The figure shows three views and two pictorial views of one solid part (mm, origin at its lowest corner). Answer the questions. Give positions to 0.01 mm unless a question says otherwise; leave off trailing zeros. Loops run counter-clockwise (first coordinate to the right, second up) from the corner with the lowest first, then second, coordinate; pieces in that order, holes last. Notation, with made-up numbers: M -36.75,89 L 21.25,89 A21 cw 21.25,117 Z; hole C -23,55.25 d2. An arc over 180 degrees is marked long. One line per item, written item: value. Start each with the question number.
Q1. Consider L1, parallel to X at y = 42.5, z = 1.7; L2, parallel to Y at x = 72.5, z = 1.65. Determine where each line is inside the solid, lowest interval first.
Q2. The mould has two halves that part along Z. Classify the marked faces 1, 2 and 3: +Z half, -Z half, draft (parallel to the pull), parting line (faces both ways), or undercut.
Q3. Flat-ended cylindrical pins translate along their axes: pin 1 (7 mm diameter, centred on x = 7.5, y = 42.5, fed in from +Z); pin 2 (8 mm diameter, centred on x = 68, z = 13, fed in from +Y); pin 3 (4 mm diameter, centred on x = 53.5, z = 34.5, fed in from +Y); pin 4 (1 mm diameter, centred on x = 38.5, y = 32, fed in from +Z). Find the tip coordinate at first contact, or state that the pin passes through.
Q4. A cutting plane is placed at B-B, the plane y = 21.5. Determine the outline of the cut face in (x, z).
Q5. A cutting plane is placed at A-A, the plane x = 40. Determine the outline of the cut face in (y, z).
Q6. A cutting plane is placed at D-D, the plane x = 29.5. Determine the outline of the cut face in (y, z), and give its area (3 significant figures).
Q7. A cutting plane is placed at C-C, the plane z = 40.5. Determine the outline of the cut face in (x, y).
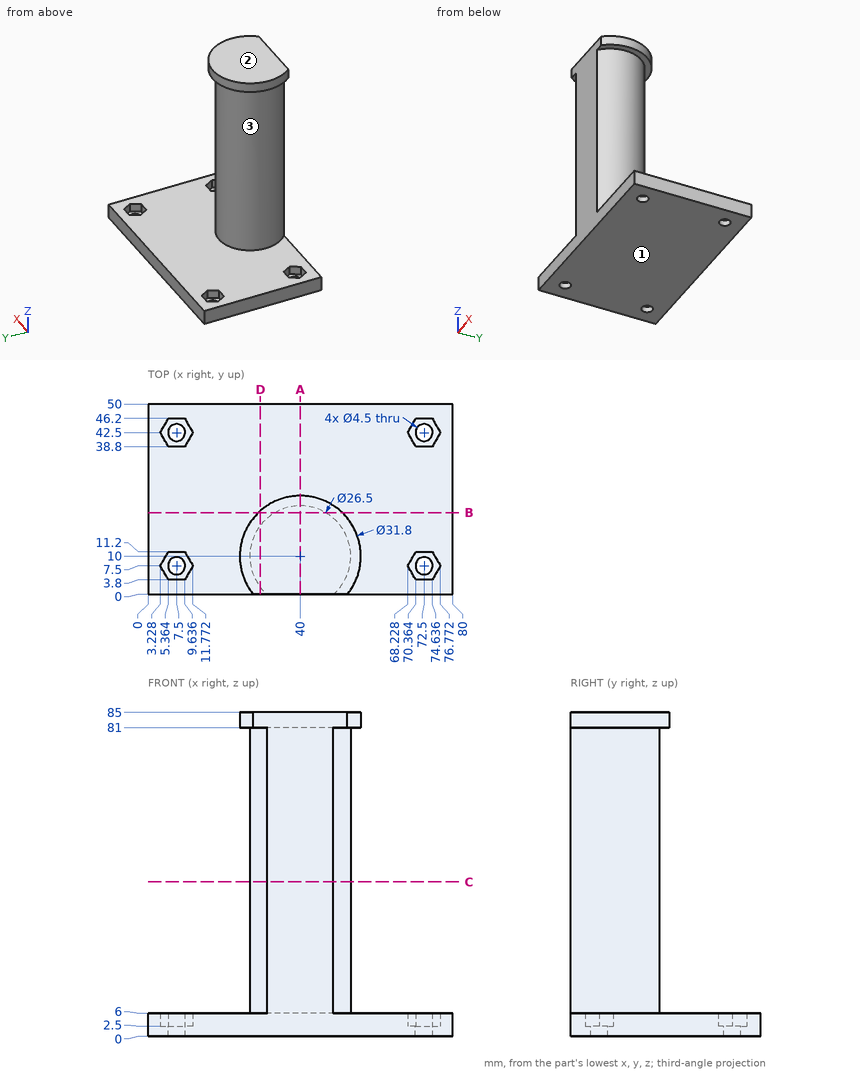
Answer block:
1. L1: 0 to 5.25, 9.75 to 70.25, 74.75 to 80
1. L2: 0 to 5.25, 9.75 to 40.25, 44.75 to 50
2. face 1: -Z half
2. face 2: +Z half
2. face 3: undercut
3. pin 1: z = 2.5
3. pin 2: through
3. pin 3: y = 16.58
3. pin 4: z = 6
4. outline: M 0,0 L 80,0 L 80,6 L 46.58,6 L 46.58,81 L 50.98,81 L 50.98,85 L 29.02,85 L 29.02,81 L 33.42,81 L 33.42,6 L 0,6 Z
5. outline: M 0,0 L 50,0 L 50,6 L 23.25,6 L 23.25,81 L 25.9,81 L 25.9,85 L 0,85 Z
6. outline: M 0,0 L 50,0 L 50,6 L 18.08,6 L 18.08,81 L 21.94,81 L 21.94,85 L 0,85 L 0,81 L 1.92,81 L 1.92,6 L 0,6 Z
6. area: 1,600 mm^2
7. outline: M 31.31,0 L 48.69,0 A13.25 ccw long Z
